For this review, take the finished solid that the model builds, in its own axes (mm). Face numbers are marked on the shaded views. Give positions to 0.01 mm unless a question says otherwise; leave off trailing zeros. Order: outer loops, then holes, each group sorted by start corner. A loop starts at its lowest first (then second) coordinate and runs counter-clockwise, first axis right, second up. Notation, with made-up numbers: M -6,29 L 30,29 A27 cw 30,61 Z; hole C -7.5,68 d2. An arc over 180 degrees is marked long. Use CSV: the item, a comma, the result in double quotes. Start each with the question number.
(1) Draft analysis for pull direction Y (two halves, no side actions). For the marked faces 1, 2 and 3, state which applies: pulls with the +Y half, pulls with the -Y half, needs draft (parallel to the pull), parting line crosses it, or undercut.
(2) Consider section A-A (y = -24). Write out the cut boundary in (x, z).
(3) Consider section C-C (x = 24.5). Write out the cut boundary in (y, z).
(4) Consider section D-D (x = 0). Give the number of separate pieces and of enclosed holes in the cut face, and give its area (3 significant figures).
(5) Consider section B-B (y = -36). Write out the cut boundary in (x, z).
(6) Clearance check with flat-ended pins moving along their axes: P1, Ø1, axis at x = 26, z = 7.5, coming from the -Y side; P2, Ø3, axis at x = -11, z = 3.5, coming from the -Y side; P3, Ø1.5, axis at y = 14, z = 7, coming from the +X side. State where each tip first meets the part, or that it passes through.
(7) Wall thickness on L1, parallel to X at y = -37, z = 5.25; L2, parallel to Y at x = -33.5, z = 5.25; L3, parallel to X at y = -23.5, z = 5.5: over which ranges is each line inside the solid? List them lowest first. Write a range as from..to.
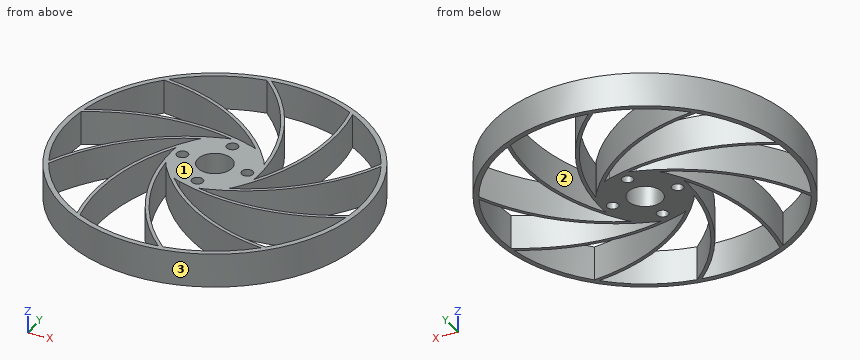
```python
from build123d import *

# Parameters (mm, degrees)
SKETCH1_R           = 44.45
SKETCH1_R_2         = 42.95
SKETCH1_R_3         = 12.7
SKETCH1_R_4         = 1.65
SKETCH1_R_5         = 5
BOSS_EXTRUDE1_DEPTH = 10


with BuildPart() as part:
    # Sketch1 → Boss-Extrude1 (new body)
    # profile 1 of 12: a face of its own
    with BuildSketch(Plane.XY):
        Circle(SKETCH1_R)
        Circle(SKETCH1_R_2, mode=Mode.SUBTRACT)
    # profile 2 of 12: a face of its own
    with BuildSketch(Plane.XY):
        with BuildLine():
            ThreePointArc((-1.742936184, 12.579832012), (1.119230316, 12.650585896), (3.924515829, 12.078417757))
            ThreePointArc((3.924515829, 12.078417757), (-19.72755965, 14.560574413), (-42.342066264, 7.20082804))
            ThreePointArc((-42.342066264, 7.20082804), (-42.445514325, 6.563597619), (-42.539372889, 5.924884318))
            ThreePointArc((-42.539372889, 5.924884318), (-22.775826214, 13.143048835), (-1.742936184, 12.579832012))
        make_face()
    # profile 3 of 12: a face of its own
    with BuildSketch(Plane.XY):
        with BuildLine():
            ThreePointArc((-8.804304726, 9.1528257), (-6.530351476, 10.892406052), (-3.924515829, 12.078417757))
            ThreePointArc((-3.924515829, 12.078417757), (-24.518421919, 0.184183522), (-38.487991711, -19.062449843))
            ThreePointArc((-38.487991711, -19.062449843), (-38.197128306, -19.638785328), (-37.897635221, -20.210683923))
            ThreePointArc((-37.897635221, -20.210683923), (-26.151320743, -2.754344892), (-8.804304726, 9.1528257))
        make_face()
    # profile 4 of 12: a face of its own
    with BuildSketch(Plane.XY):
        with BuildLine():
            ThreePointArc((-12.50272811, 2.229751063), (-11.685560963, 4.973697316), (-10.274515829, 7.464872704))
            ThreePointArc((-10.274515829, 7.464872704), (-19.944080366, -14.262559214), (-19.932812483, -38.044519796))
            ThreePointArc((-19.932812483, -38.044519796), (-19.358737547, -38.339819778), (-18.780288992, -38.626457842))
            ThreePointArc((-18.780288992, -38.626457842), (-19.537899599, -17.599672487), (-12.50272811, 2.229751063))
        make_face()
    # profile 5 of 12: a face of its own
    with BuildSketch(Plane.XY):
        with BuildLine():
            ThreePointArc((7.510489314, -42.28823773), (-5.461664877, -25.722523382), (-11.425534308, -5.545012694))
            ThreePointArc((-11.425534308, -5.545012694), (-12.377283339, -2.844794745), (-12.7, 0))
            ThreePointArc((-12.7, 0), (-7.751777987, -23.261489097), (6.236023622, -42.494876272))
            ThreePointArc((6.236023622, -42.494876272), (6.874032975, -42.396346195), (7.510489314, -42.28823773))
        make_face()
    # profile 6 of 12: a face of its own
    with BuildSketch(Plane.XY):
        with BuildLine():
            ThreePointArc((30.932515974, -29.797348129), (10.700740193, -24.020244623), (-5.98417474, -11.201770069))
            ThreePointArc((-5.98417474, -11.201770069), (-8.341304168, -9.576671905), (-10.274515829, -7.464872704))
            ThreePointArc((-10.274515829, -7.464872704), (7.401440109, -23.375320774), (30.022910658, -30.71363436))
            ThreePointArc((30.022910658, -30.71363436), (30.481156541, -30.258909364), (30.932515974, -29.797348129))
        make_face()
    # profile 7 of 12: a face of its own
    with BuildSketch(Plane.XY):
        with BuildLine():
            ThreePointArc((42.539372889, -5.924884318), (22.775826214, -13.143048835), (1.742936184, -12.579832012))
            ThreePointArc((1.742936184, -12.579832012), (-1.119230316, -12.650585896), (-3.924515829, -12.078417757))
            ThreePointArc((-3.924515829, -12.078417757), (19.72755965, -14.560574413), (42.342066264, -7.20082804))
            ThreePointArc((42.342066264, -7.20082804), (42.445514325, -6.563597619), (42.539372889, -5.924884318))
        make_face()
    # profile 8 of 12: a face of its own
    with BuildSketch(Plane.XY):
        with BuildLine():
            ThreePointArc((37.897635221, 20.210683923), (26.151320743, 2.754344892), (8.804304726, -9.1528257))
            ThreePointArc((8.804304726, -9.1528257), (6.530351476, -10.892406052), (3.924515829, -12.078417757))
            ThreePointArc((3.924515829, -12.078417757), (24.518421919, -0.184183522), (38.487991711, 19.062449843))
            ThreePointArc((38.487991711, 19.062449843), (38.197128306, 19.638785328), (37.897635221, 20.210683923))
        make_face()
    # profile 9 of 12: a face of its own
    with BuildSketch(Plane.XY):
        with BuildLine():
            ThreePointArc((18.780288992, 38.626457842), (19.537899599, 17.599672487), (12.50272811, -2.229751063))
            ThreePointArc((12.50272811, -2.229751063), (11.685560963, -4.973697316), (10.274515829, -7.464872704))
            ThreePointArc((10.274515829, -7.464872704), (19.944080366, 14.262559214), (19.932812483, 38.044519796))
            ThreePointArc((19.932812483, 38.044519796), (19.358737547, 38.339819778), (18.780288992, 38.626457842))
        make_face()
    # profile 10 of 12: a face of its own
    with BuildSketch(Plane.XY):
        with BuildLine():
            ThreePointArc((11.425534308, 5.545012694), (12.377283339, 2.844794745), (12.7, 0))
            ThreePointArc((12.7, 0), (7.751777987, 23.261489097), (-6.236023622, 42.494876272))
            ThreePointArc((-6.236023622, 42.494876272), (-6.874032975, 42.396346195), (-7.510489314, 42.28823773))
            ThreePointArc((-7.510489314, 42.28823773), (5.461664877, 25.722523382), (11.425534308, 5.545012694))
        make_face()
    # profile 11 of 12: a face of its own
    with BuildSketch(Plane.XY):
        with BuildLine():
            ThreePointArc((5.98417474, 11.201770069), (8.341304168, 9.576671905), (10.274515829, 7.464872704))
            ThreePointArc((10.274515829, 7.464872704), (-7.401440109, 23.375320774), (-30.022910658, 30.71363436))
            ThreePointArc((-30.022910658, 30.71363436), (-30.481156541, 30.258909364), (-30.932515974, 29.797348129))
            ThreePointArc((-30.932515974, 29.797348129), (-10.700740193, 24.020244623), (5.98417474, 11.201770069))
        make_face()
    # profile 12 of 12: a face of its own
    with BuildSketch(Plane.XY):
        Circle(SKETCH1_R_3)
        with Locations((-9.525, 0)):
            Circle(SKETCH1_R_4, mode=Mode.SUBTRACT)
        with Locations((9.525, 0)):
            Circle(SKETCH1_R_4, mode=Mode.SUBTRACT)
        with Locations((0, -9.525)):
            Circle(SKETCH1_R_4, mode=Mode.SUBTRACT)
        with Locations((0, 9.525)):
            Circle(SKETCH1_R_4, mode=Mode.SUBTRACT)
        Circle(SKETCH1_R_5, mode=Mode.SUBTRACT)
    extrude(amount=BOSS_EXTRUDE1_DEPTH)


solid = part.part
```
Check result:
1,face 1,"needs draft"
1,face 2,"undercut"
1,face 3,"parting line crosses it"
2,outline,"M -37.41,0 L -35.62,0 L -35.62,10 L -37.41,10 Z; M -21.15,0 L -20.15,0 L -20.15,10 L -21.15,10 Z; M -7.42,0 L -6.31,0 L -6.31,10 L -7.42,10 Z; M 8.51,0 L 10.66,0 L 10.66,10 L 8.51,10 Z; M 35.62,0 L 37.41,0 L 37.41,10 L 35.62,10 Z"
3,outline,"M -37.09,0 L -35.28,0 L -35.28,10 L -37.09,10 Z; M -29.86,0 L -28.84,0 L -28.84,10 L -29.86,10 Z; M -13.85,0 L -12.83,0 L -12.83,10 L -13.85,10 Z; M -0.2,0 L 1.15,0 L 1.15,10 L -0.2,10 Z; M 35.28,0 L 37.09,0 L 37.09,10 L 35.28,10 Z"
4,separate pieces,"10"
4,enclosed holes,"0"
4,area,"186 mm^2"
5,outline,"M -26.07,0 L -23.42,0 L -23.42,10 L -26.07,10 Z; M -20.33,0 L -19.31,0 L -19.31,10 L -20.33,10 Z; M 0.06,0 L 1.36,0 L 1.36,10 L 0.06,10 Z; M 23.42,0 L 26.07,0 L 26.07,10 L 23.42,10 Z"
6,P1,"stops at y = -36.41"
6,P2,"stops at y = -43.42"
6,P3,"stops at x = 42.43"
7,L1,"x = -24.63..-21.81, -20.15..-19.13, 0.89..2.21, 21.81..24.63"
7,L2,"y = -29.22..-26.88, -11.92..-10.1, 10.28..11.35, 26.88..29.22"
7,L3,"x = -37.73..-35.95, -21.13..-20.13, -7.64..-6.55, 7.62..9.69, 35.95..37.73"
